Build history of the part. All positions in model axes, mm. Face numbers are marked on the shaded views. A direction names the side the tool comes from. Give positions to 0.01 mm unless a question says otherwise; leave off trailing zeros. Order: outer loops, then holes, each group sorted by start corner. A loop starts at its lowest first (then second) coordinate and runs counter-clockwise, first axis right, second up. Notation, with made-up numbers: M 7.5,43.5 L 53.5,43.5 A34 ccw 53.5,78.5 Z; hole C 9.25,-22.5 d2. An arc over 180 degrees is marked long. Use CSV: the item, a comma, the result in double quotes. Start each with the question number.
Item 1: Band-saw the part on B-B on y = 19. Write the cut outline in (x, z), plus the area to 3 significant figures.
Item 2: Wall check: line 1 along Z through (x, y) = (2.5, 17); line 2 along X through (y, z) = (25.5, 6.25); line 3 along Y through (x, z) = (10.5, -10.75). Give the ranges that are in metal, low to high.
Item 3: Which spindle directions (+Z, -Z, +X, -X, +Y, -Y) get a long thin tool onto all of the face, cutting with end or side? Do the marked faces 1, 2, 3, 4 and 5. Say none if no direction does.
Item 4: Band-saw the part on A-A on z = 0. Write the cut outline in (x, y), plus the area to 3 significant figures.
Item 5: Two-plate mould, pull along X, no slides. Class the marked faces 6, 7, 8 and 9: pulls with the +X half, pulls with the -X half, needs draft (parallel to the pull), parting line crosses it, or undercut.
Item 6: Pin check, flat tips, straight feed: P1, Ø1.6, axis at x = -18.5, y = 2, coming from the +Z side; P2, Ø12, axis at x = 7.5, y = 26.5, coming from the -Z side; P3, Ø4, axis at x = -10.5, z = 9.5, coming from the -Y side; P4, Ø12, axis at y = 21, z = -5.5, coming from the +X side. Stop position of each tip, or through.
Item 7: Band-saw the part on C-C on y = 6. Write the cut outline in (x, z).
Item 8: Band-saw the part on D-D on x = 6.5. Write the cut outline in (y, z), plus the area to 3 significant figures.
Autodesk Inventor part; units mm, degrees
ref_plane "YZ Plane" through (0, 0, 0) normal (1, 0, 0) x (0, 1, 0)
ref_plane "XZ Plane" through (0, 0, 0) normal (0, 1, 0) x (-1, 0, 0)
ref_plane "XY Plane" through (0, 0, 0) normal (0, 0, 1) x (1, 0, 0)
sketch "Sketch1" plane through (0, 0, 0) normal (0, 1, 0) x (-1, 0, 0)
  line L0 (17, 15) -> (-17, 15)
  line L1 (-17, 15) -> (-17, -15)
  line L2 (-17, -15) -> (17, -15)
  line L3 (17, -15) -> (17, 15)
  line L4 (17, 15) -> (-17, -15) construction
  line L5 (-17, 15) -> (17, -15) construction
  circle A0 centre (-5, 0) radius 3
  circle A1 centre (1, 0) radius 3
  line L6 (1, 3) -> (-5, 3)
  line L7 (1, -3) -> (-5, -3)
  point P0 (0, 0)
  dimension "d0" = 34
  dimension "d1" = 30
  dimension "d2" = 6
  dimension "d3" = 12
  dimension "d4" = 6
  dimension "d5" = 18
extrude "Extrusion1" add sketch "Sketch1" along normal blind 5
sketch "Sketch2" plane through (-17, 0, -15) normal (-1, 0, 0) x (0, 0, 1)
  line L0 (30, 0) -> (0, 0)
  line L1 (0, 0) -> (30, 0)
  line L2 (30, 0) -> (30, 34)
  line L3 (30, 34) -> (0, 34)
  line L4 (0, 34) -> (0, 0)
  circle A0 centre (15, 16) radius 3
  circle A1 centre (15, 22) radius 3
  line L5 (12, 22) -> (12, 16)
  line L6 (18, 22) -> (18, 16)
  point P0 (15, 0)
  point P1 (15, 0)
  dimension "d8" = 34
  dimension "d9" = 6
  dimension "d10" = 6
  dimension "d11" = 0
  dimension "d12" = 0
  dimension "d13" = 6
  dimension "d15" = 12
extrude "Extrusion2" add sketch "Sketch2" against normal blind 5
sketch "Sketch3" plane through (17, 0, -15) normal (0, 0, -1) x (-1, 0, 0)
  line L0 (34, 34) -> (29, 34)
  line L1 (0, 5) -> (29, 34)
  line L2 (29, 34) -> (29, 5)
  line L3 (29, 5) -> (0, 5)
  point P0 (17, 0)
extrude "Extrusion3" add sketch "Sketch3" against normal blind 3
mirror "Mirror1" about plane through (0, 0, 0) normal (0, 0, 1) of "Extrusion3"
sketch "Sketch4" plane through (0, 0, 0) normal (0, -1, 0) x (1, 0, 0)
  line L0 (20, 3) -> (14, 3)
  line L1 (14, 3) -> (14, -3)
  line L2 (14, -3) -> (20, -3)
  line L3 (20, -3) -> (20, 3)
  line L4 (17, 15) -> (17, -15)
  line L5 (20, 3) -> (14, -3) construction
  line L6 (14, 3) -> (20, -3) construction
  line L7 (17, 3) -> (17, -3)
  line L8 (-20, 3) -> (-14, 3)
  line L9 (-14, 3) -> (-14, -3)
  line L10 (-14, -3) -> (-20, -3)
  line L11 (-20, -3) -> (-20, 3)
  line L12 (-17, -3) -> (-17, 3)
  line L13 (-20, 3) -> (-14, -3) construction
  line L14 (-14, 3) -> (-20, -3) construction
  line L15 (-17, 3) -> (-17, -3)
  line L16 (-17, -15) -> (-17, 15)
  point P0 (0, 0)
  point P1 (17, 0)
  point P2 (-17, 0)
  dimension "d20" = 6
  dimension "d21" = 6
  dimension "d22" = 6
  dimension "d23" = 6
extrude "Extrusion4" add sketch "Sketch4" along normal blind 4 contours L4 L2 L1 L0 | L8 L9 L10 L12
chamfer "Chamfer1" distance 1 angle 45 4 edges at (17, -2, 3) (17, -2, -3) (-17, -2, -3) (-17, -2, 3)
sketch "Sketch5" plane through (-17, 34, -15) normal (-1, 0, 0) x (0, 0, 1)
  line L0 (11, 3) -> (19, 3)
  line L1 (19, 3) -> (19, -3)
  line L2 (19, -3) -> (11, -3)
  line L3 (11, -3) -> (11, 3)
  line L4 (30, 0) -> (0, 0)
  line L5 (11, 3) -> (19, -3) construction
  line L6 (19, 3) -> (11, -3) construction
  line L7 (11, -31) -> (19, -31)
  line L8 (19, -31) -> (19, -37)
  line L9 (19, -37) -> (11, -37)
  line L10 (11, -37) -> (11, -31)
  line L11 (11, -31) -> (19, -37) construction
  line L12 (19, -31) -> (11, -37) construction
  line L13 (11, 0) -> (19, 0)
  line L14 (0, -34) -> (13, -34)
  line L15 (11, -34) -> (19, -34)
  point P0 (15, -34)
  point P1 (15, 0)
  dimension "d29" = 8
  dimension "d30" = 6
  dimension "d31" = 8
  dimension "d32" = 6
extrude "Extrusion5" add sketch "Sketch5" along normal blind 4 contours L4 L1 L2 L3 | L7 L8 L15 L14 L10
chamfer "Chamfer2" distance 1 angle 45 4 edges at (-19, 0, -4) (-19, 0, 4) (-19, 34, 4) (-19, 34, -4)
properties part number "L"
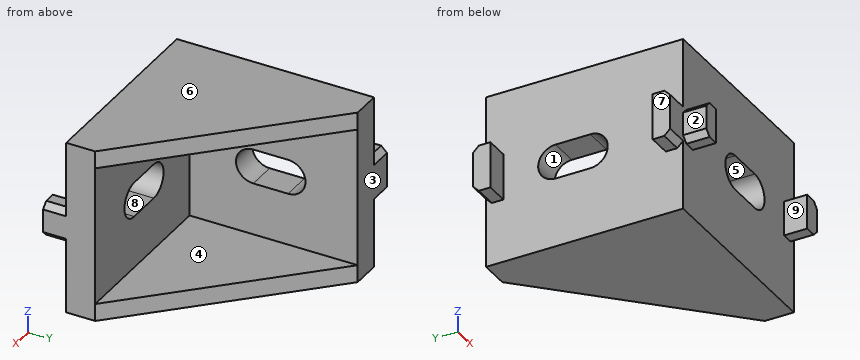
Model answer:
1,outline,"M -17,-15 L 3,-15 L 3,-12 L -12,-12 L -12,-3 L -17,-3 Z; M -17,3 L -12,3 L -12,12 L 3,12 L 3,15 L -17,15 Z"
1,area,"210 mm^2"
2,line 1,"z = -15 to -12, 12 to 15"
2,line 2,"x = -17 to -12"
2,line 3,"y = 0 to 5"
3,face 1,"+X, -X"
3,face 2,"+Z, -Z, -X, -Y"
3,face 3,"+Z, -Z, +X, -X, +Y"
3,face 4,"+X, +Y"
3,face 5,"+Y, -Y"
4,outline,"M -21,0 L -17,0 L -17,-4 L -14,-4 L -14,0 L -4,0 L -4,5 L -12,5 L -12,13 L -17,13 L -17,3 L -21,3 Z; M -21,31 L -17,31 L -17,25 L -12,25 L -12,34 L -21,34 Z; M 8,0 L 14,0 L 14,-4 L 17,-4 L 17,5 L 8,5 Z"
4,area,"243 mm^2"
5,face 6,"needs draft"
5,face 7,"pulls with the -X half"
5,face 8,"undercut"
5,face 9,"undercut"
6,P1,"stops at z = 4"
6,P2,"passes through"
6,P3,"stops at y = 0"
6,P4,"stops at x = -12"
7,outline,"M -17,-15 L 16,-15 L 16,-12 L -12,-12 L -12,12 L 16,12 L 16,15 L -17,15 Z"
8,outline,"M 0,-15 L 15.5,-15 L 15.5,-12 L 5,-12 L 5,-2.6 L 0,-2.6 Z; M 0,2.6 L 5,2.6 L 5,12 L 15.5,12 L 15.5,15 L 0,15 Z"
8,area,"187 mm^2"
